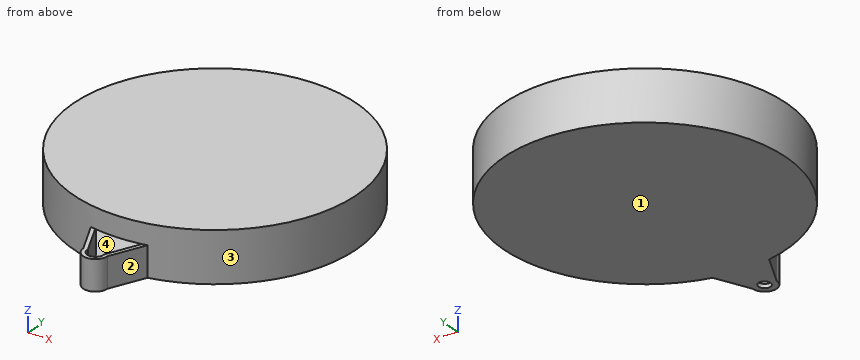
```python
from build123d import *

# Parameters (mm, degrees)
SKETCH1_R           = 70
BOSS_EXTRUDE1_DEPTH = 25
SKETCH21_R          = 6
BOSS_EXTRUDE4_DEPTH = 15
CUT_EXTRUDE2_REACH  = 118.249
SKETCH22_R          = 3
SHELL15_START       = 2
SHELL15_OUTLINE_R   = 68
SHELL15_DEPTH       = 21
SHELL15_2_OUTLINE_R = 3
SHELL15_2_DEPTH     = 13


# Read off the part's stored shape, not the designer's step: Shell15
with BuildPart() as part:
    # Sketch1 → Boss-Extrude1 (new body)
    with BuildSketch(Plane.XY):
        Circle(SKETCH1_R)
    extrude(amount=BOSS_EXTRUDE1_DEPTH)

    # Sketch21 → Boss-Extrude4 (add)
    with BuildSketch(Plane.XY):
        with Locations((0, -85.59)):
            Circle(SKETCH21_R)
        with BuildLine():
            Line((-13.97898065, -68.59), (-6, -85.59))
            ThreePointArc((-6, -85.59), (0, -79.59), (6, -85.59))
            Line((6, -85.59), (13.97898065, -68.59))
            ThreePointArc((13.97898065, -68.59), (0, -70), (-13.97898065, -68.59))
        make_face()
    extrude(amount=BOSS_EXTRUDE4_DEPTH)

    # Sketch22 → Cut-Extrude2 (cut, up to next)
    with BuildSketch(Plane.XY.offset(15), mode=Mode.PRIVATE) as cut_extrude2_sk1:
        with Locations((0, -85.59)):
            Circle(SKETCH22_R)
    cut_extrude2_tool1 = extrude(cut_extrude2_sk1.sketch, amount=-CUT_EXTRUDE2_REACH, mode=Mode.PRIVATE) & part.part
    add(cut_extrude2_tool1.solids().sort_by_distance((0, -85.59, 15))[0], mode=Mode.SUBTRACT)

    # Shell15 outline → Shell15 (cut)
    with BuildSketch(Plane.XY.offset(SHELL15_START)):
        Circle(SHELL15_OUTLINE_R)
    extrude(amount=SHELL15_DEPTH, mode=Mode.SUBTRACT)

    # Shell15 2 outline → Shell15 2 (cut)
    with BuildSketch(Plane.XY.offset(SHELL15_START)):
        with BuildLine():
            ThreePointArc((12.599173957, -66.82260707), (0, -68), (-12.599173957, -66.82260707))
            Line((-12.599173957, -66.82260707), (-3.979676533, -85.187290811))
            ThreePointArc((-3.979676533, -85.187290811), (0, -89.59), (3.979676533, -85.187290811))
            Line((3.979676533, -85.187290811), (12.599173957, -66.82260707))
        make_face()
        with Locations((0, -85.59)):
            Circle(SHELL15_2_OUTLINE_R, mode=Mode.SUBTRACT)
    extrude(amount=SHELL15_2_DEPTH, mode=Mode.SUBTRACT)


solid = part.part
```
Build history of the part. All positions in model axes, mm. Face numbers are marked on the shaded views. Give positions to 0.01 mm unless a question says otherwise; leave off trailing zeros. Loops run counter-clockwise (first coordinate to the right, second up) from the corner with the lowest first, then second, coordinate; pieces in that order, holes last.
Item 1: Drill centre lines: line 1 (Z direction, x = -31.5, y = 48.5); line 2 (Y direction, x = 0, z = 5.5); line 3 (Y direction, x = 0, z = 16). Where is each one in solid material? Low to high.
Answers follow:
line 1: z = 0 to 2, 23 to 25
line 2: y = -91.59 to -89.59, 68 to 70
line 3: y = -70 to -68, 68 to 70
Item 2: Flat gauge pins, fed straight in: pin 1 (5 mm diameter, centred on y = 44, z = 4.5, fed in from +X); pin 2 (1.6 mm diameter, centred on x = -3.5, y = -69, fed in from -Z); pin 3 (7 mm diameter, centred on x = 5, y = -82, fed in from +Z); pin 4 (12 mm diameter, centred on x = -51, z = 2.5, fed in from +Y). Where does each tip first touch, or does it go through?
Answers follow:
pin 1: stops at x = 56.37
pin 2: stops at z = 0
pin 3: stops at z = 15
pin 4: stops at y = 53.62
Item 3: Pull direction X, two halves, no side cores. Call the marked faces 1, 2, 3 and 4: released by +X, released by -X, zero draft, split by the parting line, or undercut.
Answers follow:
face 1: zero draft
face 2: released by +X
face 3: split by the parting line
face 4: undercut
Item 4: Slice it at B-B, the plane y = 0. List the corners of the cut face in (x, z).
Answers follow:
outline: (-70, 0) - (70, 0) - (70, 25) - (-70, 25) - close; hole (-68, 2) - (68, 2) - (68, 23) - (-68, 23) - close
Item 5: Slice it at C-C, the plane z = 11.75. List the corners of the cut face in (x, y), and give its area (3 significant figures).
Answers follow:
outline: (-13.98, -68.59) - (-6, -85.59) arc R6 ccw to (6, -85.59) - (13.98, -68.59) arc R70 ccw (long way) to start; hole (-12.6, -66.82) - (-3.98, -85.19) arc R4 ccw (long way) to (3.98, -85.19) - (12.6, -66.82) arc R68 ccw (long way) to start
area: 924 mm2
Item 6: Slice it at A-A, the plane x = 0. List the corners of the cut face in (y, z).
Answers follow:
outline: (-91.59, 0) - (-88.59, 0) - (-88.59, 2) - (-89.59, 2) - (-89.59, 15) - (-91.59, 15) - close; (-82.59, 0) - (70, 0) - (70, 25) - (-70, 25) - (-70, 15) - (-68, 15) - (-68, 23) - (68, 23) - (68, 2) - (-82.59, 2) - close
